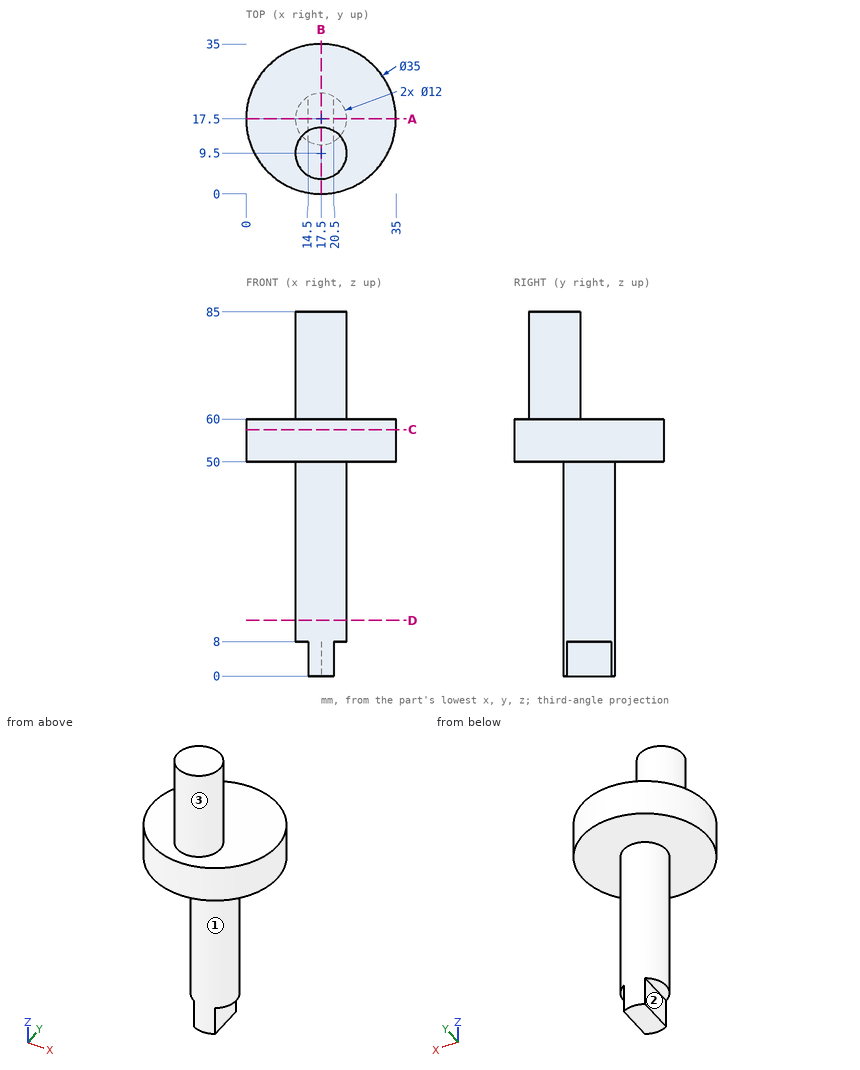
Part print with two shaded views. Sizes in mm from the minimum x, y, z corner. A direction names the side the tool comes from. Give positions to 0.01 mm unless a question says otherwise; leave off trailing zeros. Order: outer loops, then holes, each group sorted by start corner. A loop starts at its lowest first (then second) coordinate and runs counter-clockwise, first axis right, second up.
1) Saw through at B-B, the plane x = 17.5. Write the cut outline in (y, z), then the cut area to 3 significant figures.
2) Saw through at C-C, the plane z = 57.5. Write the cut outline in (x, y).
3) Pin check, flat tips, straight feed: pin 1 (12 mm diameter, centred on y = 6, z = 9, fed in from -X); pin 2 (8 mm diameter, centred on x = 26, z = 57.5, fed in from -Y); pin 3 (4 mm diameter, centred on y = 18.5, z = 2.5, fed in from -X); pin 4 (8 mm diameter, centred on y = 5.5, z = 41.5, fed in from -X). Stop position of each tip, or through.
4) Wall check: probe 1 along Z at (x, y) = (8.5, 6); probe 2 along Z at (x, y) = (22, 11.5); probe 3 along Y at (x, z) = (9.5, 58). Give the ranges that are in metal, low to high.
5) Saw through at D-D, the plane z = 13. Write the cut outline in (x, y), then the cut area to 3 significant figures.
6) 3-axis set-ups, long thin cutter, end or side, ignore diameter. For the marked faces 1, 2 and 3: which of +Z, -Z, +X, -X, +Y, -Y reach the whole face in a straight line?
7) Saw through at A-A, the plane y = 17.5. Write the cut outline in (x, z).
Computed:
1. outline: (0, 50) - (11.5, 50) - (11.5, 0) - (23.5, 0) - (23.5, 50) - (35, 50) - (35, 60) - (15.5, 60) - (15.5, 85) - (3.5, 85) - (3.5, 60) - (0, 60) - close
1. area: 1,250 mm2
2. outline: circle Ø35 at (17.5, 17.5)
3. pin 1: stops at x = 15.1
3. pin 2: stops at y = 0.59
3. pin 3: stops at x = 14.5
3. pin 4: passes through
4. probe 1: z = 50 to 60
4. probe 2: z = 50 to 85
4. probe 3: y = 1.94 to 33.06
5. outline: circle Ø12 at (17.5, 17.5)
5. area: 113 mm2
6. face 1: -Z
6. face 2: -Z, -X, +Y, -Y
6. face 3: +Z
7. outline: (0, 50) - (11.5, 50) - (11.5, 8) - (14.5, 8) - (14.5, 0) - (20.5, 0) - (20.5, 8) - (23.5, 8) - (23.5, 50) - (35, 50) - (35, 60) - (0, 60) - close
